Design review of the part shown in the three views and the two pictorial views. Dimensions are in mm from the part's minimum x, y and z. Coordinates: 2 decimals unless noted, no trailing zeros. Write each loop counter-clockwise with the first axis right and the second up, starting at its lowest first coordinate (ties: lowest second). Pieces come first, ordered by that corner, then holes.
Q1. Take a section at B-B, the plane y = 1.65. Write out the cut boundary in (x, z).
Q2. For L1, parallel to Z at x = 6.5, y = 1.25; L2, parallel to X at y = 1, z = 35 (1 decimal); L3, parallel to X at y = 0.4, z = 14 (1 decimal), list the stretches that pass through material, from the lowest coordinate up.
Q3. Take a section at A-A, the plane x = 14. Write out the cut boundary in (y, z).
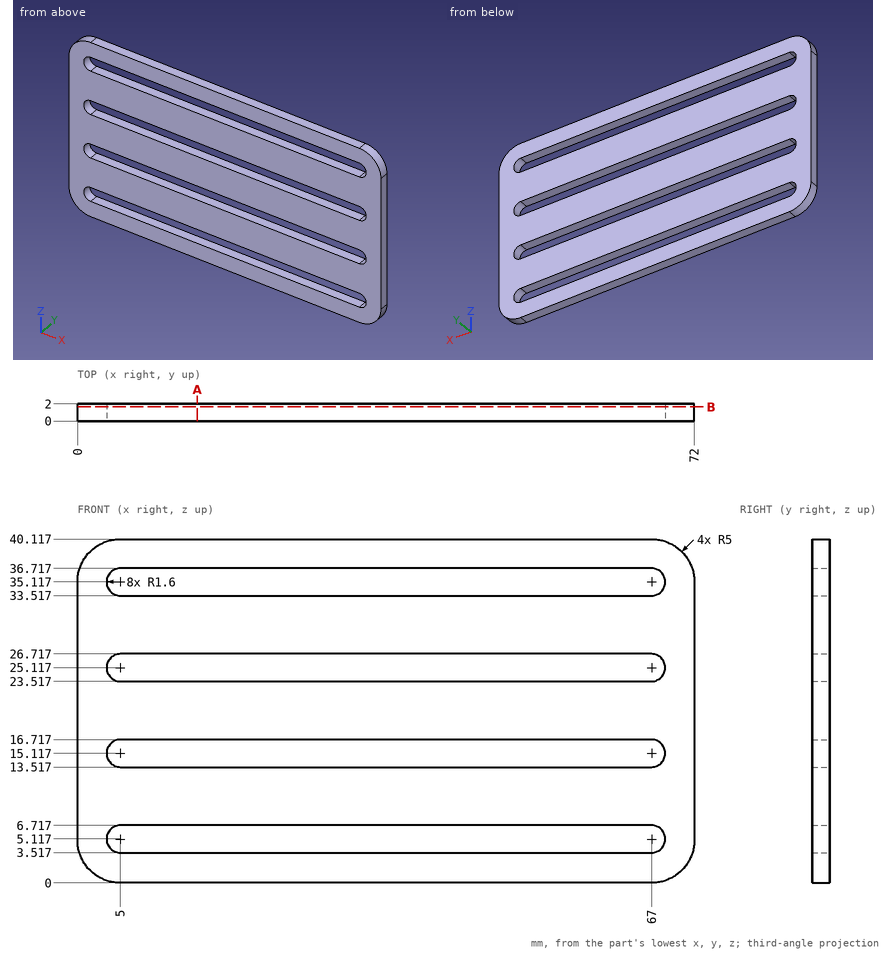
Responses:
1. outline: (0, 5) arc R5 ccw to (5, 0) - (67, 0) arc R5 ccw to (72, 5) - (72, 35.12) arc R5 ccw to (67, 40.12) - (5, 40.12) arc R5 ccw to (0, 35.12) - close; hole (5, 3.52) - (67, 3.52) arc R1.6 ccw to (67, 6.72) - (5, 6.72) arc R1.6 ccw to start; hole (5, 13.52) - (67, 13.52) arc R1.6 ccw to (67, 16.72) - (5, 16.72) arc R1.6 ccw to start; hole (5, 23.52) - (67, 23.52) arc R1.6 ccw to (67, 26.72) - (5, 26.72) arc R1.6 ccw to start; hole (5, 33.52) - (67, 33.52) arc R1.6 ccw to (67, 36.72) - (5, 36.72) arc R1.6 ccw to start
2. L1: z = 0 to 3.52, 6.72 to 13.52, 16.72 to 23.52, 26.72 to 33.52, 36.72 to 40.12
2. L2: x = 0 to 3.4, 68.6 to 72
2. L3: x = 0 to 3.9, 68.1 to 72
3. outline: (0, 0) - (2, 0) - (2, 3.52) - (0, 3.52) - close; (0, 6.72) - (2, 6.72) - (2, 13.52) - (0, 13.52) - close; (0, 16.72) - (2, 16.72) - (2, 23.52) - (0, 23.52) - close; (0, 26.72) - (2, 26.72) - (2, 33.52) - (0, 33.52) - close; (0, 36.72) - (2, 36.72) - (2, 40.12) - (0, 40.12) - close
